Could you check a few things on this model? Use its own coordinates, in mm. A direction names the side the tool comes from. Give positions to 0.01 mm unless a question says otherwise; leave off trailing zeros. Order: outer loops, then holes, each group sorted by start corner. A loop starts at its lowest first (then second) coordinate and runs counter-clockwise, first axis right, second up. Notation, with made-up numbers: (-29.75, 86) -> (-3.75, 86) arc R28 ccw to (-3.75, 124) -> close; hole circle Ø10 at (-26.75, 34.5). An arc over 180 degrees is marked (long way). Write each question's results on one line, items separated by ' | '.
Autodesk Inventor part; units mm, degrees
ref_plane "YZ Plane" through (0, 0, 0) normal (1, 0, 0) x (0, 1, 0)
ref_plane "XZ Plane" through (0, 0, 0) normal (0, 1, 0) x (-1, 0, 0)
ref_plane "XY Plane" through (0, 0, 0) normal (0, 0, 1) x (1, 0, 0)
sketch "Sketch1" plane through (0, 0, 0) normal (0, 0, 1) x (1, 0, 0)
  line L0 (0, 0) -> (52.9336, 0)
  line L1 (52.9336, 0) -> (52.9336, 114.3)
  line L2 (52.9336, 114.3) -> (0, 114.3)
  line L3 (0, 114.3) -> (0, 0)
  dimension "d0" = 114.3
  dimension "d1" = 52.9336
extrude "Extrusion1" add sketch "Sketch1" along normal blind 3.175
sketch "Sketch2" plane through (0, 0, 3.175) normal (0, 0, 1) x (1, 0, 0)
  line L0 (0, 114.3) -> (0, 0)
  line L1 (52.9336, 0) -> (52.9336, 114.3)
  line L2 (0, 60.96) -> (-3.175, 60.96)
  line L3 (-3.175, 60.96) -> (-3.175, 53.34)
  line L4 (-3.175, 53.34) -> (0, 53.34)
  line L5 (0, 53.34) -> (0, 60.96)
  line L6 (52.9336, 60.96) -> (49.7586, 60.96)
  line L7 (49.7586, 60.96) -> (49.7586, 53.34)
  line L8 (49.7586, 53.34) -> (52.9336, 53.34)
  line L9 (52.9336, 53.34) -> (52.9336, 60.96)
  line L10 (52.9336, 114.3) -> (0, 114.3)
  line L11 (0, 0) -> (52.9336, 0)
  line L12 (30.2768, 114.3) -> (22.6568, 114.3)
  line L13 (30.2768, 0) -> (30.2768, -3.175)
  line L14 (30.2768, -3.175) -> (22.6568, -3.175)
  line L15 (22.6568, -3.175) -> (22.6568, 0)
  line L16 (22.6568, 0) -> (30.2768, 0)
  line L17 (22.6568, 114.3) -> (22.6568, 111.125)
  line L18 (22.6568, 111.125) -> (30.2768, 111.125)
  line L19 (30.2768, 111.125) -> (30.2768, 114.3)
  point P0 (0, 57.15)
  point P1 (52.9336, 57.15)
  point P2 (26.4668, 114.3)
  point P3 (26.4668, 0)
  dimension "d4" = 3.81
  dimension "d5" = 7.62
  dimension "d6" = 3.175
  dimension "d7" = 3.81
  dimension "d8" = 7.62
  dimension "d9" = 3.175
  dimension "d13" = 7.62
  dimension "d14" = 3.81
  dimension "d15" = 3.175
  dimension "d20" = 7.62
  dimension "d21" = 3.81
  dimension "d22" = 3.175
extrude "Extrusion2" add sketch "Sketch2" against normal blind 3.175 contours L0 L4 L3 L2 | L10 L19 L18 L17 | L11 L13 L14 L15 | L1 L8 L7 L6
extrude "Extrusion3" cut sketch "Sketch2" against normal blind 3.175 contours L10 L19 L18 L17 | L1 L8 L7 L6
sketch "Sketch3" plane through (0, 0, 3.175) normal (0, 0, 1) x (1, 0, 0)
  line L0 (0, 60.96) -> (0, 114.3)
  line L1 (22.6568, 114.3) -> (0, 114.3)
  line L2 (0, 114.3) -> (22.6568, 114.3)
  line L3 (22.6568, 114.3) -> (22.6568, 111.125)
  line L4 (22.6568, 111.125) -> (30.2768, 111.125)
  line L5 (30.2768, 111.125) -> (22.6568, 111.125)
  line L6 (30.2768, 111.125) -> (30.2768, 114.3)
  line L7 (30.2768, 114.3) -> (52.9336, 114.3)
  line L8 (52.9336, 114.3) -> (52.9336, 60.96)
  line L9 (52.9336, 60.96) -> (52.9336, 114.3)
  line L10 (52.9336, 60.96) -> (49.7586, 60.96)
  line L11 (49.7586, 60.96) -> (49.7586, 53.34)
  line L12 (49.7586, 60.96) -> (49.7586, 53.34)
  line L13 (49.7586, 53.34) -> (52.9336, 53.34)
  line L14 (52.9336, 53.34) -> (52.9336, 0)
  line L15 (52.9336, 0) -> (52.9336, 53.34)
  line L16 (52.9336, 0) -> (30.2768, 0)
  line L17 (0, 0) -> (22.6568, 0)
  line L18 (30.2768, 0) -> (30.2768, -3.175)
  line L19 (30.2768, -3.175) -> (22.6568, -3.175)
  line L20 (22.6568, -3.175) -> (30.2768, -3.175)
  line L21 (22.6568, -3.175) -> (22.6568, 0)
  line L22 (22.6568, 0) -> (0, 0)
  line L23 (0, 0) -> (0, 53.34)
  line L24 (0, 53.34) -> (0, 0)
  line L25 (0, 53.34) -> (-3.175, 53.34)
  line L26 (-3.175, 53.34) -> (-3.175, 60.96)
  line L27 (-3.175, 60.96) -> (-3.175, 53.34)
  line L28 (-3.175, 60.96) -> (0, 60.96)
sketch "Sketch4" plane through (0, 0, 3.175) normal (0, 0, 1) x (1, 0, 0)
  circle A0 centre (26.4922, 76.2) radius 19.05
  line L0 (30.2768, 0) -> (52.9336, 0)
  line L1 (52.9336, 60.96) -> (52.9336, 114.3)
  point P0 (0, 0)
  dimension "d23" = 38.1
  dimension "d24" = 76.2
  dimension "d25" = 26.4414
sketch "Sketch5" plane through (0, 0, 3.175) normal (0, 0, 1) x (1, 0, 0)
  line L0 (6.35, 10.1986) -> (16.4034, 47.7183)
  line L1 (16.4034, 47.7183) -> (32.3606, 34.3286)
  line L2 (32.3606, 34.3286) -> (36.6232, 39.4086)
  line L3 (36.6232, 39.4086) -> (44.45, 10.1986)
  line L4 (44.45, 10.1986) -> (40.5056, 10.1986)
  line L5 (40.5056, 10.1986) -> (34.8373, 31.3529)
  line L6 (34.8373, 31.3529) -> (32.8302, 28.9609)
  line L7 (32.8302, 28.9609) -> (18.5357, 40.9555)
  line L8 (18.5357, 40.9555) -> (10.2944, 10.1986)
  line L9 (10.2944, 10.1986) -> (6.35, 10.1986)
  line L10 (0, 53.34) -> (0, 0)
  dimension "d26" = 3.81
  dimension "d27" = 3.81
  dimension "d29" = 3.81
  dimension "d31" = 75
  dimension "d32" = 38.1
  dimension "d33" = 6.35
  dimension "d34" = 75
  dimension "d35" = 3.81
  dimension "d36" = 29.21
  dimension "d38" = 65
  dimension "d39" = 5.08
extrude "Extrusion4" cut sketch "Sketch4" against normal blind 25.4
extrude "Extrusion5" cut sketch "Sketch5" against normal blind 2.54
properties part number "Birdhouse Tree Wall" material "Wood (Birch)"
Q1. I'm going to push flat-ended pins straight in: pin 1 Ø1 at (x, z) = (-1, 1.5) entering from -Y; pin 2 Ø6 at (x, y) = (22.5, 45.5) entering from -Z; pin 3 Ø1.6 at (x, z) = (38, 1) entering from -Y; pin 4 Ø1 at (y, z) = (76, 1.5) entering from -X. Where does each tip first touch, or does it pass through?
Here are the results:
pin 1: stops at y = 53.34 | pin 2: stops at z = 0 | pin 3: stops at y = 0 | pin 4: stops at x = 0
Q2. Suppose I cut it at D-D on y = 22.5. Please give me the cut outline in (x, z) (3 decimals).
Here are the results:
outline: (0, 0) -> (52.934, 0) -> (52.934, 3.175) -> (41.154, 3.175) -> (41.154, 0.635) -> (37.209, 0.635) -> (37.209, 3.175) -> (13.591, 3.175) -> (13.591, 0.635) -> (9.646, 0.635) -> (9.646, 3.175) -> (0, 3.175) -> close
Q3. For faces 5 (the flat face through (22.657, 113, 2)), 6 (the flat face through (0, 88, 2)), 7 (the flat face through (-2, 53.34, 2)), which set-ups out of +Z, -Z, +X, -X, +Y, -Y let a thin tool reach every point of the face, with its end or its side?
Here are the results:
face 5: +Z, -Z, +Y | face 6: +Z, -Z, -X, +Y | face 7: +Z, -Z, -X, -Y
Q4. Suppose I cut it at C-C on x = 24.5. Please give me the cut outline in (y, z) (3 decimals), and give its area (3 significant figures).
Here are the results:
outline: (-3.175, 0) -> (57.254, 0) -> (57.254, 3.175) -> (40.924, 3.175) -> (40.924, 0.635) -> (35.951, 0.635) -> (35.951, 3.175) -> (-3.175, 3.175) -> close; (95.146, 0) -> (111.125, 0) -> (111.125, 3.175) -> (95.146, 3.175) -> close | area: 230 mm²
Q5. Thinking about a two-plate mould opening in Y: for faces 1 (the flat face through (41, 0, 2)), 2 (the flat face through (11.306, 28.696, 1.923)), 3 (the flat face through (51, 60.96, 2)), 4 (the flat face through (42, 114.3, 2)), which applies, +Y half, -Y half, draft (parallel to the pull), parting line (faces both ways), or undercut?
Here are the results:
face 1: -Y half | face 2: undercut | face 3: undercut | face 4: +Y half
Q6. Suppose I cut it at A-A on z = 2.45. State how many separate pieces and enclosed holes the cut face has, and give its area (3 significant figures).
Here are the results:
separate pieces: 1 | enclosed holes: 2 | area: 4,580 mm²
Q7. Suppose I cut it at B-B on y = 76.2. Please give me the cut outline in (x, z) (3 decimals), and give its area (3 significant figures).
Here are the results:
outline: (0, 0) -> (7.442, 0) -> (7.442, 3.175) -> (0, 3.175) -> close; (45.542, 0) -> (52.934, 0) -> (52.934, 3.175) -> (45.542, 3.175) -> close | area: 47.1 mm²
Q8. I need wall thicknesses on line 1 along Y through (x, z) = (48, 2.95); line 2 along X through (y, z) = (2, 2.1); line 3 along Z through (x, y) = (7.5, 13.5) (3 decimals). Which ranges of each line are inside material? Lowest first, please.
Here are the results:
line 1: y = 0 to 114.3 | line 2: x = 0 to 52.93 | line 3: z = 0 to 0.635
